Source: CAD feature listing. Evaluate the final solid. Frame: model axes, mm. A direction names the side the tool comes from. Give positions to 0.01 mm unless a question says otherwise; leave off trailing zeros. Loops run counter-clockwise (first coordinate to the right, second up) from the corner with the lowest first, then second, coordinate; pieces in that order, holes last. Notation, with made-up numbers: (-2, 24) -> (46, 24) arc R9 ccw to (46, 37) -> close; hole circle Ø5 at (32, 82). An arc over 180 degrees is marked (long way). Answer as a JSON object with one key per item and string values. Group by question number.
Autodesk Inventor part; units mm, degrees
ref_plane "YZ Plane" through (0, 0, 0) normal (1, 0, 0) x (0, 1, 0)
ref_plane "XZ Plane" through (0, 0, 0) normal (0, 1, 0) x (-1, 0, 0)
ref_plane "XY Plane" through (0, 0, 0) normal (0, 0, 1) x (1, 0, 0)
sketch "Sketch1" plane through (0, 0, 0) normal (0, 0, 1) x (1, 0, 0)
  circle A0 centre (-66.446, -8.2221) radius 2.0955
  arc A1 (-69.8715, -4.9134) -> (-69.0877, -12.1847) centre (-66.446, -8.2221) ccw
  circle A2 centre (-39.4585, 19.7179) radius 2.0955
  circle A3 centre (-1.3585, 19.7179) radius 2.0955
  arc A4 (-39.4585, 24.4804) -> (-42.884, 23.0266) centre (-39.4585, 19.7179) ccw
  arc A5 (0.8155, 23.9553) -> (-1.3585, 24.4804) centre (-1.3585, 19.7179) ccw
  line L0 (-39.4585, 24.4804) -> (-1.3585, 24.4804)
  line L1 (-69.8715, -4.9134) -> (-42.884, 23.0266)
  circle A6 centre (-52.1585, -17.7471) radius 2.0955
  arc A7 (-54.8002, -21.7097) -> (-52.1585, -22.5096) centre (-52.1585, -17.7471) ccw
  circle A8 centre (-20.4085, -17.7471) radius 2.0955
  circle A9 centre (8.1665, -17.7471) radius 2.0955
  circle A10 centre (71.6665, -17.7471) radius 2.0955
  arc A11 (71.6665, -22.5096) -> (73.8405, -13.5097) centre (71.6665, -17.7471) ccw
  line L2 (0.8155, 23.9553) -> (73.8405, -13.5097)
  line L3 (-52.1585, -22.5096) -> (71.6665, -22.5096)
  line L4 (-54.8002, -21.7097) -> (-69.0877, -12.1847)
  line L5 (-28.575, 14.3204) -> (-37.1677, 14.3204)
  line L6 (-53.5722, -10.3176) -> (-50.5242, -12.3496)
  line L7 (-19.456, -12.3496) -> (-22.504, -10.3176)
  line L8 (-10.6535, -12.3496) -> (-13.7015, -10.3176)
  line L9 (-13.7015, -10.3176) -> (45.361, -10.3176)
  line L10 (-13.7015, -10.3176) -> (45.361, -10.3176) construction
  line L11 (-44.45, -12.3496) -> (-19.456, -12.3496)
  line L12 (-10.6535, -12.3496) -> (49.3216, -12.3496)
  line L13 (-50.5242, -12.3496) -> (-47.6187, -10.3176)
  line L14 (-44.45, -12.3496) -> (-43.0953, -10.3176)
  line L15 (-53.5722, -10.3176) -> (-47.6187, -10.3176)
  line L16 (-43.0953, -10.3176) -> (-22.504, -10.3176)
  line L17 (-53.5722, -10.3176) -> (-47.6187, -10.3176) construction
  line L18 (-43.0953, -10.3176) -> (-22.504, -10.3176) construction
  line L19 (-55.6904, -4.856) -> (-50.4835, -8.3613)
  line L20 (-51, 0) -> (-45.7931, -3.5053)
  line L21 (-49.0715, 1.9965) -> (-43.8646, -1.5088)
  line L22 (-50.4835, -8.3613) -> (-45.7931, -3.5053)
  line L23 (-43.8646, -1.5088) -> (-28.575, 14.3204)
  line L24 (-37.1677, 14.3204) -> (-49.0715, 1.9965)
  line L25 (-51, 0) -> (-55.6904, -4.856)
  line L26 (-2.6623, 14.3204) -> (-2.6623, 6.2412)
  line L27 (-2.6623, 6.2412) -> (23.3297, 0.9854)
  line L28 (23.3297, 0.9854) -> (-2.6623, 14.3204)
  line L29 (49.3216, -12.3496) -> (45.361, -10.3176)
  line L30 (-6.0786, 14.3204) -> (-18.313, 11.1125)
  line L31 (-18.313, 11.1125) -> (-25.4, 0)
  line L32 (-25.4, 0) -> (-19.456, -8.3613)
  line L33 (-19.456, -8.3613) -> (-14.5251, -4.856)
  line L34 (-14.5251, -4.856) -> (-18.6777, 0.9854)
  line L35 (-18.6777, 0.9854) -> (-14.5251, 7.4968)
  line L36 (-14.5251, 7.4968) -> (-6.0786, 9.9421)
  line L37 (-6.0786, 9.9421) -> (-6.0786, 14.3204)
  point P0 (0, 0)
  dimension "d0" = 9.525
  dimension "d1" = 9.525
  dimension "d2" = 9.525
  dimension "d3" = 9.525
  dimension "d4" = 4.191
  dimension "d5" = 4.191
  dimension "d6" = 9.525
  dimension "d9" = 10.16
extrude "Extrusion1" add sketch "Sketch1" along normal blind 1.5875
equation "\"BendRadius\" = Thickness"
equation "\"BendReliefWidth\" = Thickness"
equation "\"BendReliefDepth\" = 0.5 * Thickness"
equation "\"CornerReliefSize\" = 4 * Thickness"
equation "\"MinimumRemnant\" = 2 * Thickness"
equation "\"TransitionRadius\" = BendRadius"
equation "\"JacobiRadiusSize\" = BendRadius"
equation "\"GapSize\" = Thickness"
properties part number "battery_mount_plate" material "Acetal Resin, White"
(1) Section query B-B on z = 0.7. State how many separate pieces and enclosed holes the cut face has, plus the area to 3 significant figures.
(2) Mould query, pull axis X, two halves, no side actions, for faces 1 (the face through (36.817, 5.485, 0.783)), 2 (the face through (-56.57, 8.86, 0.78)), 3 (the face through (-53.1, -6.6, 0.8)). Classes: pulls with the +X half, pulls with the -X half, needs draft (parallel to the pull), parting line crosses it, or undercut.
(3) First-contact query: pin 1 (0.5 mm diameter, centred on y = 12.5, z = 1, fed in from -X); pin 2 (0.5 mm diameter, centred on x = 23, z = 1, fed in from +Y). Flat tips, straight axial feed; report the tip coordinate or a pass-through.
(4) Section query A-A on y = 5. Return the cut outline in (x, z), plus the area to 3 significant figures.
(5) Access query for faces 4 (the face through (-36.33, 6.29, 0.78)), 5 (the face through (2, -4, 0)). Directions: +Z, -Z, +X, -X, +Y, -Y. A direction counts if a zero-diameter tool reaches every point of the face in a straight line with its end or side. Return the directions, or none.
(6) Material intervals for line 1 (Y direction, x = -4.5, z = 1.2); line 2 (X direction, y = -11, z = 0.1); line 3 (Y direction, x = 6, z = 0.8), sorted ascending. Write a range as from..to.
Result:
{
 "1": {"separate pieces": "1", "enclosed holes": "14", "area": "4,170 mm²"},
 "2": {"face 1": "pulls with the +X half", "face 2": "pulls with the -X half", "face 3": "undercut"},
 "3": {"pin 1": "x = -53.29", "pin 2": "y = 12.7"},
 "4": {"outline": "(-60.3, 0) -> (-46.17, 0) -> (-46.17, 1.59) -> (-60.3, 1.59) -> close; (-37.58, 0) -> (-22.21, 0) -> (-22.21, 1.59) -> (-37.58, 1.59) -> close; (-16.12, 0) -> (3.48, 0) -> (3.48, 1.59) -> (-16.12, 1.59) -> close; (15.5, 0) -> (37.76, 0) -> (37.76, 1.59) -> (15.5, 1.59) -> close", "area": "113 mm²"},
 "5": {"face 4": "+Z, -Z", "face 5": "-Z, +X, -X, +Y, -Y"},
 "6": {"line 1": "-22.51..-12.35, -10.32..24.48", "line 2": "-70.31..-52.55, -48.59..-43.55, -21.48..-12.68, 46.69..68.95", "line 3": "-22.51..-12.35, -10.32..4.49, 9.88..21.3"}
}
